Could you check a few things on this model? Use its own coordinates, in mm. A direction names the side the tool comes from. Coordinates: 2 decimals unless noted, no trailing zeros. Write each loop counter-clockwise with the first axis right and the second up, starting at its lowest first coordinate (ties: lowest second). Pieces come first, ordered by that corner, then holes. Notation, with made-up numbers: (34, -10.75) - (55, -10.75) arc R17 ccw to (55, 15.25) - close; hole circle Ø2 at (67.5, -27.5). An arc over 180 degrees is marked (long way). Answer as a JSON object with one key per item and string values. Group by question number.
1) If we section it at C-C (y = 1.1): Write out the boundary of the cut face in (x, z).
2) If we section it at B-B (z = 0): Write out the boundary of the cut face in (x, y).
3) On a 3-axis mill with a long thin cutter (end or side, diameter ignored), from which of +Z, -Z, +X, -X, +Y, -Y can I reach the whole of each face in a straight line? I mean faces 4 (the flat face through (-1.65, 1, 0)), 5 (the flat face through (-3, 2, 0)). Say none if no direction works.
4) We'd pull the mould along Z, two halves only. Please class faces 1 (the cylindrical face through (4.89, 1.01, -0.02)), 2 (the flat face through (-3, 0, 0)), 3 (the cylindrical face through (1.802, 1.746, 5.723)): released by +Z, released by -Z, zero draft, split by the parting line, or undercut.
5) Please list where these lines run through material, in increasing order: line 1 along Y through (x, z) = (5.75, 1.5); line 2 along Z through (x, y) = (1, 1.3); line 3 along Z through (x, y) = (3.5, 0.35).
6) Will this pin go through, and if not, where does the flat tip stop? pin 1 Ø0.6 at (y, z) = (1, -0.5) entering from +X.
7) If we section it at A-A (x = 0): Write out the boundary of the cut face in (y, z), plus the area to 3 significant figures.
```python
from build123d import *

# Parameters (mm, degrees)
SKIZZE1_R                       = 6
AUFSATZ_LINEAR_AUSTRAGEN1_DEPTH = 2
SKIZZE3_W                       = 3.3
SKIZZE3_H                       = 3.3
SCHNITT_LINEAR_AUSTRAGEN1_DEPTH = 3
SKIZZE4_R                       = 1.15
SCHNITT_LINEAR_AUSTRAGEN2_DEPTH = 3


with BuildPart() as part:
    # Skizze1 → Aufsatz-Linear austragen1 (new body)
    with BuildSketch(Plane(origin=(0, 0, 0), x_dir=(1, 0, 0), z_dir=(0, 1, 0))):
        with Locations(Location((0, 0, 0), (0, 0, 270))):
            Circle(SKIZZE1_R)
    extrude(amount=AUFSATZ_LINEAR_AUSTRAGEN1_DEPTH)

    # Skizze3 → Schnitt-Linear austragen1 (cut)
    with BuildSketch(Plane(origin=(0, 2, 0), x_dir=(1, 0, 0), z_dir=(0, 1, 0))):
        Rectangle(SKIZZE3_W, SKIZZE3_H)
    extrude(amount=-SCHNITT_LINEAR_AUSTRAGEN1_DEPTH, mode=Mode.SUBTRACT)

    # Skizze4 → Schnitt-Linear austragen2 (cut)
    with BuildSketch(Plane(origin=(0, 2, 0), x_dir=(1, 0, 0), z_dir=(0, 1, 0))):
        with Locations(Location((3.75, -0.126446108, 0), (0, 0, 270))):
            Circle(SKIZZE4_R)
    extrude(amount=-SCHNITT_LINEAR_AUSTRAGEN2_DEPTH, mode=Mode.SUBTRACT)

    # Skizze6 → Schnitt-Rotation2 (revolve, cut)
    with BuildSketch(Plane.XY, mode=Mode.PRIVATE) as schnitt_rotation2_sk:
        with BuildLine():
            Line((-6, 1.5), (-6, 0.5))
            ThreePointArc((-6, 0.5), (-5.384840005, 1), (-6, 1.5))
        make_face()
    revolve(schnitt_rotation2_sk.sketch.rotate(Axis((0, 2, 0), (0, -1, 0)), 270), axis=Axis((0, 2, 0), (0, -1, 0)), mode=Mode.SUBTRACT)


solid = part.part
```
Here are the results:
{
 "1": {"outline": "circle Ø10.79 at (0, 0); hole (-1.65, -1.65) - (1.65, -1.65) - (1.65, 1.65) - (-1.65, 1.65) - close; hole circle Ø2.3 at (3.75, 0.13)"},
 "2": {"outline": "(-6, 0) - (-1.65, 0) - (-1.65, 2) - (-6, 2) - (-6, 1.5) arc R0.51 cw (long way) to (-6, 0.5) - close; (1.65, 0) - (2.61, 0) - (2.61, 2) - (1.65, 2) - close; (4.89, 0) - (6, 0) - (6, 0.5) arc R0.51 cw (long way) to (6, 1.5) - (6, 2) - (4.89, 2) - close"},
 "3": {"face 4": "+Y, -Y", "face 5": "+Z, -Z, +X, -X, +Y"},
 "4": {"face 1": "undercut", "face 2": "zero draft", "face 3": "split by the parting line"},
 "5": {"line 1": "y = 0 to 0.49, 1.51 to 2", "line 2": "z = -5.39 to -1.65, 1.65 to 5.39", "line 3": "z = -4.87 to -1, 1.25 to 4.87"},
 "6": {"pin 1": "stops at x = 5.46"},
 "7": {"outline": "(0, -6) - (0.5, -6) arc R0.51 cw (long way) to (1.5, -6) - (2, -6) - (2, -1.65) - (0, -1.65) - close; (0, 1.65) - (2, 1.65) - (2, 6) - (1.5, 6) arc R0.51 cw (long way) to (0.5, 6) - (0, 6) - close", "area": "16.4 mm²"}
}
